Source: CAD feature listing. Evaluate the final solid. Frame: model axes, mm. A direction names the side the tool comes from. Round coordinates to 2 decimals unless told otherwise and drop trailing zeros. Loops run counter-clockwise (first coordinate to the right, second up) from the corner with the lowest first, then second, coordinate; pieces in that order, holes last. Notation, with made-up numbers: M -32,9.25 L -19,9.25 A19 cw -19,37.25 Z; hole C 20,13 d2. An arc over 180 degrees is marked long. One line per item, written item: value.
from build123d import *

# Parameters (mm, degrees)
SKETCH2_W                                           = 69.85
SKETCH2_H                                           = 44.45
BOSS_EXTRUDE1_DEPTH                                 = 4.7752
CUT_EXTRUDE1_DEPTH                                  = 1
CUT_EXTRUDE1_DEPTH_BACK                             = 45.45
CHAMFER1_SIZE                                       = 0.762
CSK_FOR_1_4_FLAT_HEAD_MACHINE_SCREW_100_D           = 6.7564
CSK_FOR_1_4_FLAT_HEAD_MACHINE_SCREW_100_DEPTH       = 4.826
CSK_FOR_1_4_FLAT_HEAD_MACHINE_SCREW_100_CSINK_D     = 12.8778
CSK_FOR_1_4_FLAT_HEAD_MACHINE_SCREW_100_CSINK_ANGLE = 100
CSK_FOR_1_4_FLAT_HEAD_MACHINE_SCREW_100_TIP         = 2.029827343


with BuildPart() as part:
    # Sketch2 → Boss-Extrude1 (new body)
    with BuildSketch(Plane(origin=(0, 0, 0), x_dir=(1, 0, 0), z_dir=(0, 1, 0))):
        with Locations((1.080982686, -0.881944444)):
            Rectangle(SKETCH2_W, SKETCH2_H)
    extrude(amount=BOSS_EXTRUDE1_DEPTH)

    # Sketch3 → Cut-Extrude1 (cut, two sides)
    with BuildSketch(Plane(origin=(0, 0, -21.343055556), x_dir=(-1, 0, 0), z_dir=(0, 0, -1))) as cut_extrude1_sk:
        Polygon((-0.888710757, 2.3876), (-3.463824269, -0.187513512), (1.686402756, -0.187513512), align=None)
    extrude(amount=CUT_EXTRUDE1_DEPTH, mode=Mode.SUBTRACT)
    extrude(cut_extrude1_sk.sketch, amount=-CUT_EXTRUDE1_DEPTH_BACK, mode=Mode.SUBTRACT)

    # Chamfer1
    chamfer1_edges = [part.edges().sort_by_distance(p)[0] for p in [
        (-17.671453278, 0, -21.343055556),
        (19.641146722, 0, 23.106944444),
        (19.641146722, 0, -21.343055556),
        (36.005982686, 0, 0.881944444),
        (-17.671453278, 0, 23.106944444),
        (-33.844017314, 0, 0.881944444),
    ]]
    chamfer(chamfer1_edges, length=CHAMFER1_SIZE)

    # CSK for 1/4 Flat Head Machine Screw (100)1
    with Locations(Plane(origin=(0, 0, 0), x_dir=(-1, 0, 0), z_dir=(0, -1, 0))):
        with Locations((-20.130982686, 2.293055556), (17.969017314, 2.293055556)):
            CounterSinkHole(CSK_FOR_1_4_FLAT_HEAD_MACHINE_SCREW_100_D / 2, CSK_FOR_1_4_FLAT_HEAD_MACHINE_SCREW_100_CSINK_D / 2, depth=CSK_FOR_1_4_FLAT_HEAD_MACHINE_SCREW_100_DEPTH, counter_sink_angle=CSK_FOR_1_4_FLAT_HEAD_MACHINE_SCREW_100_CSINK_ANGLE)
            with Locations((0, 0, -(CSK_FOR_1_4_FLAT_HEAD_MACHINE_SCREW_100_DEPTH + CSK_FOR_1_4_FLAT_HEAD_MACHINE_SCREW_100_TIP / 2))):  # 118° drill point
                Cone(0, CSK_FOR_1_4_FLAT_HEAD_MACHINE_SCREW_100_D / 2, CSK_FOR_1_4_FLAT_HEAD_MACHINE_SCREW_100_TIP, mode=Mode.SUBTRACT)


solid = part.part
1. Reachability of faces 4 (the face through (-33.844, 3, 1)), 5 (the face through (-0.3, 1.2, 0.6)) from +Z, -Z, +X, -X, +Y, -Y: full face, straight path, thin tool, end or side. Return the list, or none.
Report:
face 4: +Z, -Z, -X, +Y, -Y
face 5: +Z, -Z, -Y
2. Section query A-A (y = 1.7). Return the cut outline in (x, z), and give its area (3 significant figures).
Report:
outline: M -33.84,-21.34 L 0.2,-21.34 L 0.2,23.11 L -33.84,23.11 Z; M 1.58,-21.34 L 36.01,-21.34 L 36.01,23.11 L 1.58,23.11 Z; hole C -17.97,-2.29 d8.83; hole C 20.13,-2.29 d8.83
area: 2,920 mm2
3. Section query D-D (x = 0). Return the cut outline in (y, z).
Report:
outline: M 1.5,-21.34 L 4.78,-21.34 L 4.78,23.11 L 1.5,23.11 Z
4. Pin query (flat end, axial travel): pin 1 (8 mm diameter, centred on x = 20.13, z = -2.29, fed in from -Y). Return the tip coordinate at first contact, or that it passes through.
Report:
pin 1: stops at y = 2.04
5. Ray query, line 1 (X direction, y = 3.7, z = -5); line 2 (X direction, y = 1.45, z = 1); line 3 (X direction, y = 0.3, z = -5.5). Return the intervals inside material, ascending. Write a range as [from, to].
Report:
line 1: x = [-33.84, -19.99], [-15.95, 18.11], [22.15, 36.01]
line 2: x = [-33.84, -21.34], [-14.6, -0.05], [1.83, 16.76], [23.5, 36.01]
line 3: x = [-33.38, -23.14], [-12.8, -1.2], [2.98, 14.96], [25.3, 35.54]
6. Pull-direction query (X, two-part tool) for faces 1 (the face through (36.006, 3, 1)), 2 (the face through (19, 0, 5)), 3 (the face through (-14.71, 2.44, -0.94)); classes: released by +X, released by -X, zero draft, split by the parting line, or undercut.
Report:
face 1: released by +X
face 2: zero draft
face 3: undercut
7. Section query B-B (z = 17). Return the cut outline in (x, y).
Report:
outline: M -33.84,0.76 L -33.08,0 L -1.5,0 L 0.89,2.39 L 3.28,0 L 35.24,0 L 36.01,0.76 L 36.01,4.78 L -33.84,4.78 Z
8. Section query C-C (z = -3). Count the separate pieces of the cut face and the enclosed holes in it, and give its area (3 significant figures).
Report:
separate pieces: 3
enclosed holes: 0
area: 248 mm2
